Could you check a few things on this model? Use its own coordinates, in mm. A direction names the side the tool comes from. Coordinates: 2 decimals unless noted, no trailing zeros. Write each loop counter-clockwise with the first axis right and the second up, starting at its lowest first coordinate (ties: lowest second). Pieces come first, ordered by that corner, then holes. Notation, with made-up numbers: (73.5, -31.75) - (88.5, -31.75) arc R30 cw to (88.5, -9.75) - close; hole circle Ø6 at (85.5, -13.5). An arc over 180 degrees is marked (long way). Answer as a JSON object with one key per item and string values. Group by question number.
1) If we section it at B-B (x = -1.5): Write out the boundary of the cut face in (y, z), plus the area to 3 significant figures.
2) On a 3-axis mill with a long thin cutter (end or side, diameter ignored), from which of +Z, -Z, +X, -X, +Y, -Y can I reach the whole of each face in a straight line? I mean faces 5 (the cylindrical face through (0.9, 4.51, 2.86)), 6 (the cylindrical face through (-1.802, 0.507, 5.723)), 7 (the cylindrical face through (-2, 2, 0)). Say none if no direction works.
3) If we section it at D-D (x = 5): Write out the boundary of the cut face in (y, z), plus the area to 3 significant figures.
4) We'd pull the mould along Z, two halves only. Please class faces 1 (the flat face through (-2, 5, 1)), 2 (the flat face through (3, 4, 1)), 3 (the cylindrical face through (-0.9, 0.51, 2.86)), 4 (the cylindrical face through (-3.955, 2.465, -5.158)): released by +Z, released by -Z, zero draft, split by the parting line, or undercut.
5) If we section it at A-A (z = 0): Write out the boundary of the cut face in (x, y), plus the area to 3 significant figures.
6) If we section it at C-C (z = -2.5): Write out the boundary of the cut face in (x, y).
7) Please list where these lines run through material, in increasing order: line 1 along X through (y, z) = (0.5, 0); line 2 along X through (y, z) = (2.85, 0); line 3 along X through (y, z) = (4.7, -1.5).
8) Will this pin go through, and if not, where does the flat tip stop? pin 1 Ø2 at (y, z) = (3.5, 3) entering from +X.
```python
from build123d import *

# Parameters (mm, degrees)
SKETCH_1_R          = 6.5
SKETCH_1_R_2        = 2
EXTRUDE_1_DEPTH     = 5
SKETCH_2_R          = 6
SKETCH_2_R_2        = 3
CUT_EXTRUDE_1_DEPTH = 1
CUT_EXTRUDE_START   = -1
SKETCH_3_R          = 6
SKETCH_3_R_2        = 3
CUT_EXTRUDE_2_DEPTH = 1


with BuildPart() as part:
    # Эскиз1 → Бобышка-Вытянуть1 (new body)
    with BuildSketch(Plane(origin=(0, 0, 0), x_dir=(1, 0, 0), z_dir=(0, 1, 0))):
        with Locations(Location((0, 0, 0), (0, 0, 270))):
            Circle(SKETCH_1_R)
        with Locations(Location((0, 0, 0), (0, 0, 270))):
            Circle(SKETCH_1_R_2, mode=Mode.SUBTRACT)
    extrude(amount=EXTRUDE_1_DEPTH)

    # Эскиз2 → Вырез-Вытянуть1 (cut)
    with BuildSketch(Plane(origin=(0, 5, 0), x_dir=(1, 0, 0), z_dir=(0, 1, 0))):
        with Locations(Location((0, 0, 0), (0, 0, 270))):
            Circle(SKETCH_2_R)
        with Locations(Location((0, 0, 0), (0, 0, 270))):
            Circle(SKETCH_2_R_2, mode=Mode.SUBTRACT)
    extrude(amount=-CUT_EXTRUDE_1_DEPTH, mode=Mode.SUBTRACT)

    # Эскиз3 → Вырез-Вытянуть2 (cut)
    with BuildSketch(Plane.XZ.offset(CUT_EXTRUDE_START)):
        with Locations(Location((0, 0, 0), (0, 0, 90))):
            Circle(SKETCH_3_R)
        with Locations(Location((0, 0, 0), (0, 0, 90))):
            Circle(SKETCH_3_R_2, mode=Mode.SUBTRACT)
    extrude(amount=CUT_EXTRUDE_2_DEPTH, mode=Mode.SUBTRACT)


solid = part.part
```
Here are the results:
{
 "1": {"outline": "(0, -6.32) - (5, -6.32) - (5, -5.81) - (4, -5.81) - (4, -2.6) - (5, -2.6) - (5, -1.32) - (0, -1.32) - (0, -2.6) - (1, -2.6) - (1, -5.81) - (0, -5.81) - close; (0, 1.32) - (5, 1.32) - (5, 2.6) - (4, 2.6) - (4, 5.81) - (5, 5.81) - (5, 6.32) - (0, 6.32) - (0, 5.81) - (1, 5.81) - (1, 2.6) - (0, 2.6) - close", "area": "37.2 mm²"},
 "2": {"face 5": "+Y", "face 6": "-Y", "face 7": "+Y, -Y"},
 "3": {"outline": "(0, -4.15) - (5, -4.15) - (5, -3.32) - (4, -3.32) - (4, 3.32) - (5, 3.32) - (5, 4.15) - (0, 4.15) - (0, 3.32) - (1, 3.32) - (1, -3.32) - (0, -3.32) - close", "area": "28.3 mm²"},
 "4": {"face 1": "zero draft", "face 2": "undercut", "face 3": "undercut", "face 4": "split by the parting line"},
 "5": {"outline": "(-6.5, 0) - (-6, 0) - (-6, 1) - (-3, 1) - (-3, 0) - (-2, 0) - (-2, 5) - (-3, 5) - (-3, 4) - (-6, 4) - (-6, 5) - (-6.5, 5) - close; (2, 0) - (3, 0) - (3, 1) - (6, 1) - (6, 0) - (6.5, 0) - (6.5, 5) - (6, 5) - (6, 4) - (3, 4) - (3, 5) - (2, 5) - close", "area": "33.0 mm²"},
 "6": {"outline": "(-6, 0) - (-5.45, 0) - (-5.45, 1) - (-1.66, 1) - (-1.66, 0) - (1.66, 0) - (1.66, 1) - (5.45, 1) - (5.45, 0) - (6, 0) - (6, 5) - (5.45, 5) - (5.45, 4) - (1.66, 4) - (1.66, 5) - (-1.66, 5) - (-1.66, 4) - (-5.45, 4) - (-5.45, 5) - (-6, 5) - close"},
 "7": {"line 1": "x = -6.5 to -6, -3 to -2, 2 to 3, 6 to 6.5", "line 2": "x = -6.5 to -2, 2 to 6.5", "line 3": "x = -6.32 to -5.81, -2.6 to -1.32, 1.32 to 2.6, 5.81 to 6.32"},
 "8": {"pin 1": "stops at x = 6.18"}
}
